from build123d import *

# Parameters (mm, degrees)
F0_W     = 400
F0_H     = 762
F1_DEPTH = 12
F2_W     = 6
F2_H     = 762
F3_DEPTH = 6
F4_W     = 6
F4_H     = 762
F5_DEPTH = 6
F6_W     = 388
F6_H     = 6
F7_DEPTH = 6
F8_W     = 388
F8_H     = 6
F9_DEPTH = 6


with BuildPart() as f1:
    # F0 (on Top) → F1 (new body)
    with BuildSketch(Plane.XY):
        Rectangle(F0_W, F0_H)
    extrude(amount=F1_DEPTH)

    # F2 (on face) → F3 (cut)
    with BuildSketch(Plane.XY.offset(12)):
        with Locations((-197, 0)):
            Rectangle(F2_W, F2_H)
    extrude(amount=-F3_DEPTH, mode=Mode.SUBTRACT)

    # F4 (on face) → F5 (cut)
    with BuildSketch(Plane.XY.offset(12)):
        with Locations((197, 0)):
            Rectangle(F4_W, F4_H)
    extrude(amount=-F5_DEPTH, mode=Mode.SUBTRACT)

    # F6 (on face) → F7 (cut)
    with BuildSketch(Plane.XY.offset(12)):
        with Locations((0, 378)):
            Rectangle(F6_W, F6_H)
    extrude(amount=-F7_DEPTH, mode=Mode.SUBTRACT)

    # F8 (on face) → F9 (cut)
    with BuildSketch(Plane.XY.offset(12)):
        with Locations((0, -378)):
            Rectangle(F8_W, F8_H)
    extrude(amount=-F9_DEPTH, mode=Mode.SUBTRACT)


solid = f1.part
Can you work these out from the model? Positions are in its coordinate system, mm. Give positions to 0.01 mm unless a question says otherwise; leave off trailing zeros. Loops run counter-clockwise (first coordinate to the right, second up) from the corner with the lowest first, then second, coordinate; pieces in that order, holes last. Notation, with made-up numbers: (-33, 60.5) - (-21, 60.5) arc R17 ccw to (-21, 76.5) - close; hole circle Ø4 at (57.5, 47). An arc over 180 degrees is marked (long way). Answer as a JSON object with one key per item and string values.
Q1. Will these pins go through, and if not, where does the flat tip stop? P1, Ø6.5, axis at y = -28.5, z = 9.5, coming from the +X side; P2, Ø1.8, axis at y = -41, z = 9.5, coming from the -X side; P3, Ø5, axis at x = -24, z = 9, coming from the -Y side.
Geometry says:
{"P1": "x = 194", "P2": "x = -194", "P3": "y = -375"}
Q2. If I drill on L1, parallel to X at y = -126.5, z = 11.75; L2, parallel to Y at x = 147, z = 7.25, over which ranges is the centre line in solid material (lowest first)?
Geometry says:
{"L1": "-194 to 194", "L2": "-375 to 375"}
Q3. Imagine slicing it at A-A on z = 9. Write out the boundary of the cut face in (x, y), plus the area to 3 significant figures.
Geometry says:
{"outline": "(-194, -375) - (194, -375) - (194, 375) - (-194, 375) - close", "area": "291,000 mm²"}
